from build123d import *

# Parameters (mm, degrees)
MAIN_EXTRUSION_DEPTH            = 30
ESQUISSE2_W                     = 19
ESQUISSE2_H                     = 10
EXTERNAL_HOLE_DEPTH             = 37.986484018
ESQUISSE3_R                     = 1.6
MAKERBEAMFIXINGHOLE_DEPTH       = 38.815340802
ESQUISSE4_R                     = 1.5
HOLELINKWITHCODERSSUPPORT_DEPTH = 27.702059846
CONG_2_R                        = 2
CONG_3_R                        = 5
ESQUISSE6_R                     = 2.5
ESQUISSE6_R_2                   = 1.5
BOSS_EXTRU_1_DEPTH              = 0.5
ESQUISSE7_R                     = 2.5
ESQUISSE7_R_2                   = 1.5
BOSS_EXTRU_2_DEPTH              = 0.5


with BuildPart() as part:
    # Esquisse1 → Main Extrusion (new body)
    with BuildSketch(Plane.XY):
        Polygon((-11, 13), (-11, -5), (11, -5), (11, -1.45), (12, -1.45), (12, 1.45), (11, 1.45), (11, 13), align=None)
    extrude(amount=MAIN_EXTRUSION_DEPTH)

    # Esquisse2 → External Hole (cut, through all)
    with BuildSketch(Plane(origin=(0, 13, 0), x_dir=(1, 0, 0), z_dir=(0, 1, 0))):
        with Locations((-1.5, -5)):
            Rectangle(ESQUISSE2_W, ESQUISSE2_H)
        with Locations((-1.5, -25)):
            Rectangle(ESQUISSE2_W, ESQUISSE2_H)
    extrude(amount=-EXTERNAL_HOLE_DEPTH, mode=Mode.SUBTRACT)

    # Esquisse3 → MakerBeamFixingHole (cut, through all)
    with BuildSketch(Plane.ZY.offset(-8)):
        with Locations(Location((5, 0, 0), (0, 0, 270))):
            Circle(ESQUISSE3_R)
        with Locations(Location((25, 0, 0), (0, 0, 270))):
            Circle(ESQUISSE3_R)
    extrude(amount=-MAKERBEAMFIXINGHOLE_DEPTH, mode=Mode.SUBTRACT)

    # Esquisse4 → HoleLinkWithCodersSupport (cut, through all)
    with BuildSketch(Plane.XY.offset(20)):
        with Locations((-3, 4)):
            Circle(ESQUISSE4_R)
    extrude(amount=-HOLELINKWITHCODERSSUPPORT_DEPTH, mode=Mode.SUBTRACT)

    # Congé2
    cong_2_edges = [part.edges().sort_by_distance(p)[0] for p in [
        (8, 4, 10),
        (8, 4, 20),
    ]]
    fillet(cong_2_edges, radius=CONG_2_R)

    # Congé3
    cong_3_edges = [part.edges().sort_by_distance(p)[0] for p in [
        (-11, 13, 15),
        (-11, -5, 15),
    ]]
    fillet(cong_3_edges, radius=CONG_3_R)

    # Esquisse6 → Boss.-Extru.1 (add)
    with BuildSketch(Plane(origin=(0, 0, 10), x_dir=(-1, 0, 0), z_dir=(0, 0, -1))):
        with Locations(Location((3, 4, 0), (0, 0, 180))):
            Circle(ESQUISSE6_R)
        with Locations(Location((3, 4, 0), (0, 0, 180))):
            Circle(ESQUISSE6_R_2, mode=Mode.SUBTRACT)
    extrude(amount=BOSS_EXTRU_1_DEPTH)

    # Esquisse7 → Boss.-Extru.2 (add)
    with BuildSketch(Plane.XY.offset(20)):
        with Locations((-3, 4)):
            Circle(ESQUISSE7_R)
        with Locations((-3, 4)):
            Circle(ESQUISSE7_R_2, mode=Mode.SUBTRACT)
    extrude(amount=BOSS_EXTRU_2_DEPTH)


solid = part.part
Can you work these out from the model? Positions are in its coordinate system, mm. A direction names the side the tool comes from. Give positions to 0.01 mm unless a question says otherwise; leave off trailing zeros. Order: outer loops, then holes, each group sorted by start corner. A loop starts at its lowest first (then second) coordinate and runs counter-clockwise, first axis right, second up. Notation, with made-up numbers: M 25,80 L 56,80 A18 cw 56,94 Z; hole C 7,-13.5 d3. An arc over 180 degrees is marked long. Use one line per item in the form item = value. Start each with the question number.
Item 1: If we section it at A-A (z = 5): Write out the boundary of the cut face in (x, y).
Item 2: Will these pins go through, and if not, where does the flat tip stop? pin 1 Ø2.5 at (y, z) = (1, 24) entering from -X; pin 2 Ø8.5 at (x, y) = (-6, 6.5) entering from +Z; pin 3 Ø10 at (x, z) = (-2.5, 4) entering from +Y; pin 4 Ø4 at (y, z) = (10.5, 22.5) entering from +X.
Item 3: For faces 1 (the flat face through (-1, 6, 20)), 2 (the flat face through (11, 7, 15)), 3 (the flat face through (11.5, -1.45, 2.1)), which set-ups out of +Z, -Z, +X, -X, +Y, -Y let a thin tool reach every point of the face, with its end or its side?
Item 4: We'd pull the mould along Z, two halves only. Please class faces 4 (the flat face through (10, 4, 30)), 5 (the flat face through (10, 4, 0)), 6 (the cylindrical face through (9.97, 1.6, 5.07)), 7 (the flat face through (4, -5, 15)): +Z half, -Z half, draft (parallel to the pull), parting line (faces both ways), or undercut.
Item 5: If we section it at C-C (x = -3): Write out the boundary of the cut face in (y, z).
Item 6: If I drill on line 1 along Z through (x, y) = (10.7, 0); line 2 along X through (y, z) = (4, 17.75); line 3 along Y through (x, z) = (10.3, 5), over which ranges is the centre line in solid material (lowest first)?
Item 7: If we section it at B-B (y = 4): Write out the boundary of the cut face in (x, z), then the cut area to 3 significant figures.
Item 8: If we section it at D-D (z = 28.25): Write out the boundary of the cut face in (x, y), then the cut area to 3 significant figures.
Outcome:
q1.outline = M 8,-5 L 11,-5 L 11,-1.6 L 8,-1.6 Z; M 8,1.6 L 11,1.6 L 11,13 L 8,13 Z
q2.pin_1 = 8
q2.pin_2 = 20.5
q2.pin_3 = through
q2.pin_4 = 11
q3.face_1 = +Z
q3.face_2 = +Z, -Z, +X, +Y
q3.face_3 = +Z, -Z, +X, -Y
q4.face_4 = +Z half
q4.face_5 = -Z half
q4.face_6 = undercut
q4.face_7 = draft
q5.outline = M -5,10 L 1.5,10 L 1.5,9.5 L 2.5,9.5 L 2.5,20.5 L 1.5,20.5 L 1.5,20 L -5,20 Z; M 5.5,9.5 L 6.5,9.5 L 6.5,10 L 13,10 L 13,20 L 6.5,20 L 6.5,20.5 L 5.5,20.5 Z
q6.line_1 = 0 to 3.4, 6.6 to 23.4, 26.6 to 30
q6.line_2 = -11 to -4.5, -1.5 to 11
q6.line_3 = -5 to -1.6, 1.6 to 13
q7.outline = M -11,10 L -5.5,10 L -5.5,9.5 L -4.5,9.5 L -4.5,20.5 L -5.5,20.5 L -5.5,20 L -11,20 Z; M -1.5,9.5 L -0.5,9.5 L -0.5,10 L 6,10 A2 cw 8,8 L 8,0 L 11,0 L 11,30 L 8,30 L 8,22 A2 cw 6,20 L -0.5,20 L -0.5,20.5 L -1.5,20.5 Z
q7.area = 254 mm2
q8.outline = M 8,-5 L 11,-5 L 11,-1.45 L 12,-1.45 L 12,1.45 L 11,1.45 L 11,13 L 8,13 Z
q8.area = 56.9 mm2
